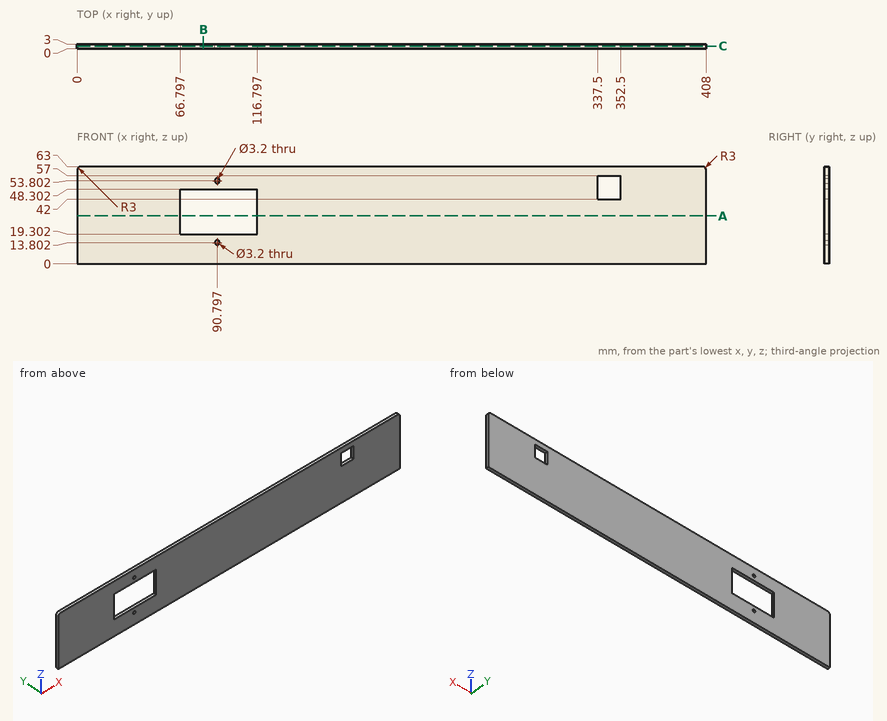
Geometry check sheet. Reference: drawing and pictorial views, mm from the part's lowest x, y, z. Round coordinates to 2 decimals unless told otherwise and drop trailing zeros. Loops run counter-clockwise (first coordinate to the right, second up) from the corner with the lowest first, then second, coordinate; pieces in that order, holes last. Notation, with made-up numbers: (88, 0) - (145, 0) arc R14 ccw to (145, 19) - close; hole circle Ø10 at (-33.5, 88.25). An arc over 180 degrees is marked (long way). Use a Markdown table: item, result. Add a question column.
1. Section check A-A, the plane z = 31. Record the boundary of the cut face in (x, y), plus the area to 3 significant figures.
2. Section check C-C, the plane y = 1.55. Record the boundary of the cut face in (x, z).
3. Section check B-B, the plane x = 82. Record the boundary of the cut face in (y, z), plus the area to 3 significant figures.
4. Thickness scan on probe 1 along X at (y, z) = (0.9, 44); probe 2 along Z at (x, y) = (351, 0.55); probe 3 along X at (y, z) = (0.9, 35). Record the ranges inside material, lowest first. Write a range as [from, to].
Checks:
| question | item | result |
|---|---|---|
| 1 | outline | (0, 0) - (66.8, 0) - (66.8, 3) - (0, 3) - close; (116.8, 0) - (408, 0) - (408, 3) - (116.8, 3) - close |
| 1 | area | 1,070 mm^2 |
| 2 | outline | (0, 0) - (408, 0) - (408, 60) arc R3 ccw to (405, 63) - (3, 63) arc R3 ccw to (0, 60) - close; hole (66.8, 19.3) - (116.8, 19.3) - (116.8, 48.3) - (66.8, 48.3) - close; hole circle Ø3.2 at (90.8, 13.8); hole circle Ø3.2 at (90.8, 53.8); hole (337.5, 42) - (352.5, 42) - (352.5, 57) - (337.5, 57) - close |
| 3 | outline | (0, 0) - (3, 0) - (3, 19.3) - (0, 19.3) - close; (0, 48.3) - (3, 48.3) - (3, 63) - (0, 63) - close |
| 3 | area | 102 mm^2 |
| 4 | probe 1 | x = [0, 66.8], [116.8, 337.5], [352.5, 408] |
| 4 | probe 2 | z = [0, 42], [57, 63] |
| 4 | probe 3 | x = [0, 66.8], [116.8, 408] |
